The model under review builds one solid part; all positions refer to its coordinate system, in mm. A direction names the side the tool comes from. Round coordinates to 2 decimals unless told otherwise and drop trailing zeros. Write each loop counter-clockwise with the first axis right and the second up, starting at its lowest first coordinate (ties: lowest second). Pieces come first, ordered by that corner, then holes. Notation, with made-up numbers: (-36.5, -27.75) -> (-25.5, -27.75) arc R13 cw to (-25.5, -12.75) -> close; hole circle Ø11 at (2.25, 76.5). An arc over 180 degrees is marked (long way). Answer in a Markdown table with one row per item. Add a question column.
```python
from build123d import *

# Parameters (mm, degrees)
F4_D     = 5
F4_DEPTH = 25


with BuildPart() as f1:
    # F0 (on Front) → F1 (revolve)
    with BuildSketch(Plane.XZ):
        Polygon((0, 6), (0, 0), (105, 0), (105, 6), (87.52, 6), (87.52, 5.35), (86.5, 5.35), (86.5, 6), (76.5, 6), (76.5, 10), (28.5, 10), (28.5, 6), (18.5, 6), (18.5, 5.35), (17.48, 5.35), (17.48, 6), align=None)
    revolve(axis=Axis((52.5, 0, 0), (1, 0, 0)))

    # F4
    with Locations(Plane.XZ.offset(6)):
        with Locations((6, 0), (99, 0)):
            Hole(F4_D / 2, depth=F4_DEPTH)


solid = f1.part
```
1. Insertion check: pin 1 Ø1 at (x, z) = (56, 7) entering from -Y; pin 2 Ø5 at (x, y) = (46.5, 7) entering from -Z; pin 3 Ø1 at (x, y) = (63.5, 7) entering from -Z. Each pin has a flat end and moves straight along its axis. Give the tip position at first contact, or say it passes through.
2. Add section B-B on x = 24. Write out the cut boundary in (y, z).
3. Tool access review of faces 1 (the cylindrical face through (52.16, 9.76, -2.17)), 2 (the cylindrical face through (96.14, 2.3, 5.54)), 3 (the flat face through (28.5, 0, 7)), 4 (the cylindrical face through (17.983, 5.223, -1.16)): name each direction out of +Z, -Z, +X, -X, +Y, -Y from which nothing blocks a thin tool from reaching the whole face with its end or side.
4. Add section A-A on y = 0. State how many separate pieces and enclosed holes the cut face has, plus the area to 3 significant figures.
5. For L1, parallel to X at y = -2, z = 0; L2, parallel to X at y = 0.25, z = -1.25; L3, parallel to X at y = -6, z = 4, list the stretches that pass through material, from the lowest coordinate up.
6. Mouldability with a two-part tool opening along X and no side actions: class faces 5 (the cylindrical face through (23, 0, -6)), 6 (the flat face through (105, 0, 0)), 7 (the cylindrical face through (101, 0.1, -1.5)) as pulls with the +X half, pulls with the -X half, needs draft (parallel to the pull), parting line crosses it, or undercut.
Filled in:
| question | item | result |
|---|---|---|
| 1 | pin 1 | y = -7.6 |
| 1 | pin 2 | z = -8.93 |
| 1 | pin 3 | z = -7.6 |
| 2 | outline | circle Ø12 at (0, 0) |
| 3 | face 1 | +X, -X |
| 3 | face 2 | +X |
| 3 | face 3 | -X |
| 3 | face 4 | none |
| 4 | separate pieces | 1 |
| 4 | enclosed holes | 2 |
| 4 | area | 1,600 mm² |
| 5 | L1 | 0 to 3.5, 8.5 to 96.5, 101.5 to 105 |
| 5 | L2 | 0 to 3.83, 8.17 to 96.83, 101.17 to 105 |
| 5 | L3 | 28.5 to 76.5 |
| 6 | face 5 | needs draft |
| 6 | face 6 | pulls with the +X half |
| 6 | face 7 | undercut |
